from build123d import *

# Parameters (mm, degrees)
BOSS_EXTRUDE2_DEPTH = 8
BOSS_EXTRUDE3_DEPTH = 23
SKETCH6_R           = 1.55
CUT_EXTRUDE1_DEPTH  = 31


with BuildPart() as part:
    # Sketch1 → Boss-Extrude2 (new body)
    with BuildSketch(Plane.XY):
        with BuildLine():
            Line((72.5875, 25.569607814), (24.291666667, 49.344857184))
            ThreePointArc((24.291666667, 49.344857184), (-55, 0), (24.291666667, -49.344857184))
            Line((24.291666667, -49.344857184), (72.5875, -25.569607814))
            ThreePointArc((72.5875, -25.569607814), (88.5, 0), (72.5875, 25.569607814))
        make_face()
    extrude(amount=BOSS_EXTRUDE2_DEPTH)

    # Sketch5 → Boss-Extrude3 (add)
    with BuildSketch(Plane.XY.offset(8)):
        with BuildLine():
            Line((20.758333333, 42.167423412), (69.054166667, 18.392174041))
            ThreePointArc((69.054166667, 18.392174041), (80.5, 0), (69.054166667, -18.392174041))
            Line((69.054166667, -18.392174041), (20.758333333, -42.167423412))
            ThreePointArc((20.758333333, -42.167423412), (-47, 0), (20.758333333, 42.167423412))
        make_face()
        with BuildLine():
            Line((65.520833333, 11.214740269), (17.225, 34.98998964))
            ThreePointArc((17.225, 34.98998964), (-39, 0), (17.225, -34.98998964))
            Line((17.225, -34.98998964), (65.520833333, -11.214740269))
            ThreePointArc((65.520833333, -11.214740269), (72.5, 0), (65.520833333, 11.214740269))
        make_face(mode=Mode.SUBTRACT)
    extrude(amount=BOSS_EXTRUDE3_DEPTH)

    # Sketch6 → Cut-Extrude1 (cut)
    with BuildSketch(Plane.XY.offset(31)):
        with Locations((0, 43)):
            Circle(SKETCH6_R)
        with Locations((-30.405591591, 30.405591591)):
            Circle(SKETCH6_R)
        with Locations((-43, 0)):
            Circle(SKETCH6_R)
        with Locations((-30.405591591, -30.405591591)):
            Circle(SKETCH6_R)
        with Locations((0, -43)):
            Circle(SKETCH6_R)
        with Locations((76.5, 0)):
            Circle(SKETCH6_R)
        with Locations((58.315707785, 19.220123822)):
            Circle(SKETCH6_R)
        with Locations((32.44935499, 31.953706526)):
            Circle(SKETCH6_R)
        with Locations((58.315707785, -19.220123822)):
            Circle(SKETCH6_R)
        with Locations((32.44935499, -31.953706526)):
            Circle(SKETCH6_R)
    extrude(amount=-CUT_EXTRUDE1_DEPTH, mode=Mode.SUBTRACT)


solid = part.part
The listing builds one solid part. Answer for the finished solid, in the listing's coordinates (mm). A direction names the side the tool comes from. Round coordinates to 2 decimals unless told otherwise and drop trailing zeros. Order: outer loops, then holes, each group sorted by start corner. A loop starts at its lowest first (then second) coordinate and runs counter-clockwise, first axis right, second up. Notation, with made-up numbers: (-38.75, -33.75) -> (-27.75, -33.75) arc R19 ccw to (-27.75, -12.75) -> close; hole circle Ø9 at (23, -18). An arc over 180 degrees is marked (long way). Write each question's results on one line, items separated by ' | '. Start each with the question number.
Q1. The mould has two halves that part along Y. Classify faces 1 (the cylindrical face through (80.498, 0.32, 19.339)), 2 (the cylindrical face through (59.794, 19.686, 15.717)), 3 (the flat face through (45.244, -30.113, 19.339)), 4 (the cylindrical face through (72.5, -0.2, 19.3)): pulls with the +Y half, pulls with the -Y half, needs draft (parallel to the pull), parting line crosses it, or undercut.
Q2. Which of the six approach directions +Z, -Z, +X, -X, +Y, -Y give full straight-line access (tool end or side, diameter ignored) to faces 5 (the cylindrical face through (-38.984, 1.107, 19.339)), 6 (the flat face through (48.78, 37.29, 3.94)), 7 (the flat face through (44.568, 30.446, 19.339))?
Q3. Find section A-A (x = 0). Determine the outline of the cut face in (y, z), then the cut area to 3 significant figures.
Q4. Find section D-D (z = 10). Give the number of separate pieces and of enclosed holes in the cut face, then the cut area to 3 significant figures.
Q5. Each of these flat-tipped pins is pushed along its axis until it touches: pin 1 (3 mm diameter, centred on y = -30.5, z = 14.5, fed in from +X); pin 2 (10 mm diameter, centred on x = -20.5, z = 15.5, fed in from -Y); pin 3 (10 mm diameter, centred on y = 27.5, z = 17.5, fed in from -X). Where does it stop, or does it pass through?
Q6. Find section B-B (y = 0). Determine the outline of the cut face in (x, z).
Q7. Straight lines are drawn through the part: probe 1 along Y at (x, z) = (0, 20); probe 2 along Y at (x, z) = (32, 14.5); probe 3 along X at (y, z) = (-18.5, 8.5). For each, find the intervals that lie inside material, in ascending order. Write a range as from..to.
Q8. Find section C-C (x = -43). Determine the outline of the cut face in (y, z), then the cut area to 3 significant figures.
Worked answers:
1) face 1: parting line crosses it | face 2: undercut | face 3: pulls with the -Y half | face 4: undercut
2) face 5: +Z | face 6: +Z, -Z, +X, +Y | face 7: +Z, +X, +Y
3) outline: (-55, 0) -> (-44.55, 0) -> (-44.55, 31) -> (-47, 31) -> (-47, 8) -> (-55, 8) -> close; (-41.45, 0) -> (41.45, 0) -> (41.45, 31) -> (39, 31) -> (39, 8) -> (-39, 8) -> (-39, 31) -> (-41.45, 31) -> close; (44.55, 0) -> (55, 0) -> (55, 8) -> (47, 8) -> (47, 31) -> (44.55, 31) -> close | area: 1,060 mm2
4) separate pieces: 1 | enclosed holes: 11 | area: 2,480 mm2
5) pin 1: stops at x = 47.51 | pin 2: stops at y = -44.37 | pin 3: stops at x = -41.26
6) outline: (-55, 0) -> (-44.55, 0) -> (-44.55, 31) -> (-47, 31) -> (-47, 8) -> (-55, 8) -> close; (-41.45, 0) -> (74.95, 0) -> (74.95, 31) -> (72.5, 31) -> (72.5, 8) -> (-39, 8) -> (-39, 31) -> (-41.45, 31) -> close; (78.05, 0) -> (88.5, 0) -> (88.5, 8) -> (80.5, 8) -> (80.5, 31) -> (78.05, 31) -> close
7) probe 1: y = -47..-44.55, -41.45..-39, 39..41.45, 44.55..47 | probe 2: y = -36.63..-33.44, -30.47..-27.72, 27.72..30.47, 33.44..36.63 | probe 3: x = -43.21..-34.33, 50.72..56.94, 59.69..68.84
8) outline: (-34.29, 0) -> (-1.55, 0) -> (-1.55, 31) -> (-18.97, 31) -> (-18.97, 8) -> (-34.29, 8) -> close; (1.55, 0) -> (34.29, 0) -> (34.29, 8) -> (18.97, 8) -> (18.97, 31) -> (1.55, 31) -> close | area: 1,330 mm2
